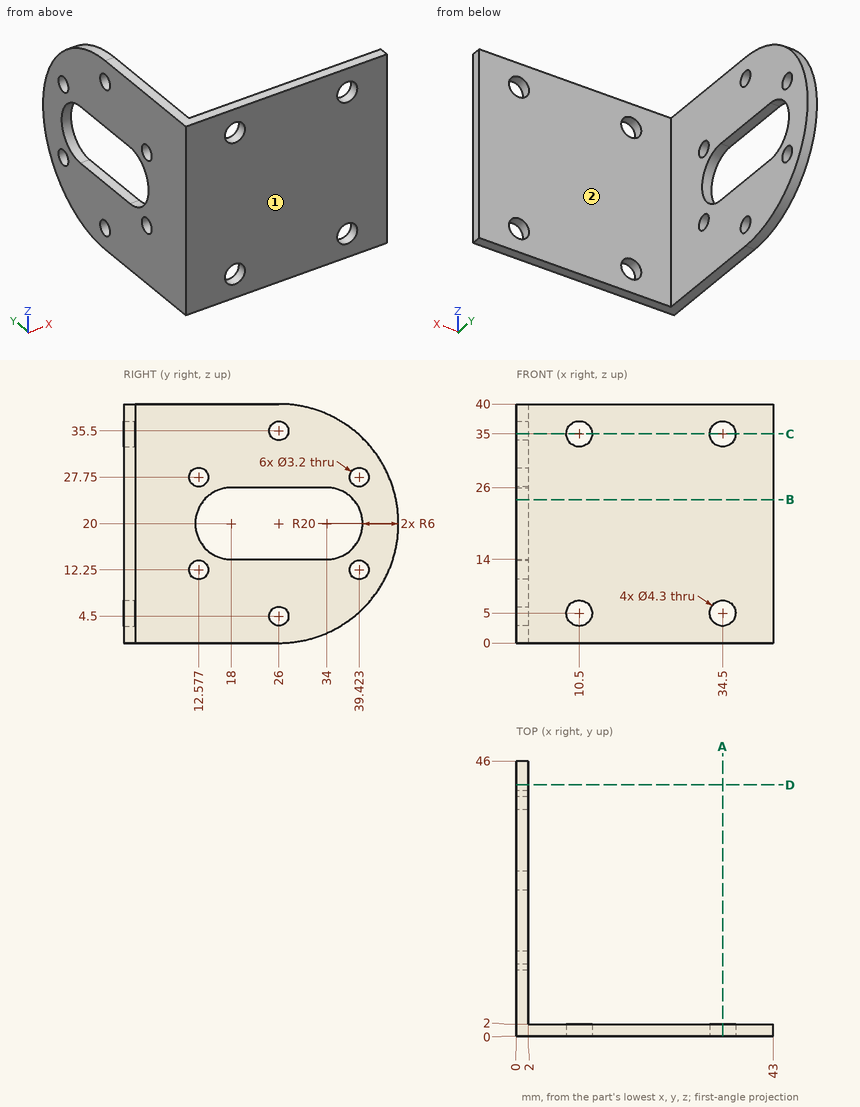
For this review, use the dimensioned drawing (mm, ordinates from the lowest corner) and the shaded views. A direction names the side the tool comes from. Round coordinates to 2 decimals unless told otherwise and drop trailing zeros. Write each loop counter-clockwise with the first axis right and the second up, starting at its lowest first coordinate (ties: lowest second). Pieces come first, ordered by that corner, then holes. Notation, with made-up numbers: (5.5, 10) - (16.5, 10) arc R23 ccw to (16.5, 37) - close; hole circle Ø8 at (75.5, 60). An arc over 180 degrees is marked (long way). One line per item, written item: value. Start each with the question number.
1. Consider section D-D on y = 42. Write out the cut boundary in (x, z), and give its area (3 significant figures).
2. To check wall thickness, follow L1, parallel to X at y = 0.95, z = 5; L2, parallel to Y at x = 0.75, z = 27.75; L3, parallel to Z at x = 10, y = 1. State the ranges of each line that lie inside material, in increasing order. Write a range as from..to.
3. Consider section B-B on z = 24. Write out the cut boundary in (x, y), and give its area (3 significant figures).
4. Consider section A-A on x = 34.5. Write out the cut boundary in (y, z).
5. Consider section C-C on z = 35. Write out the cut boundary in (x, y).
6. Clearance check with flat-ended pins moving along their axes: P1, Ø5, axis at x = 29, z = 33.5, coming from the +Y side; P2, Ø5, axis at y = 26, z = 7, coming from the +X side; P3, Ø1, axis at x = 1, y = 28.5, coming from the +Z side. State where each tip first meets the part, or that it passes through.
7. Machinability: for the marked faces 1 and 2, which of the approach directions +Z, -Z, +X, -X, +Y, -Y give a long, thin tool a straight path to every point of the face, cutting with its end or side? Answer none if there is none.
Checks:
1. outline: (0, 8) - (2, 8) - (2, 32) - (0, 32) - close
1. area: 48.0 mm^2
2. L1: x = 0..8.35, 12.65..32.35, 36.65..43
2. L2: y = 0..10.98, 14.18..37.82, 41.02..44.44
2. L3: z = 0..2.91, 7.09..32.91, 37.09..40
3. outline: (0, 0) - (43, 0) - (43, 2) - (2, 2) - (2, 13.53) - (0, 13.53) - close; (0, 38.47) - (2, 38.47) - (2, 45.6) - (0, 45.6) - close
3. area: 123 mm^2
4. outline: (0, 0) - (2, 0) - (2, 2.85) - (0, 2.85) - close; (0, 7.15) - (2, 7.15) - (2, 32.85) - (0, 32.85) - close; (0, 37.15) - (2, 37.15) - (2, 40) - (0, 40) - close
5. outline: (0, 0) - (8.35, 0) - (8.35, 2) - (2, 2) - (2, 24.48) - (0, 24.48) - close; (0, 27.52) - (2, 27.52) - (2, 39.23) - (0, 39.23) - close; (12.65, 0) - (32.35, 0) - (32.35, 2) - (12.65, 2) - close; (36.65, 0) - (43, 0) - (43, 2) - (36.65, 2) - close
6. P1: stops at y = 2
6. P2: stops at x = 2
6. P3: stops at z = 39.9
7. face 1: +Z, -Z, +X, -X, -Y
7. face 2: +Z, -Z, +X, +Y
